Autodesk Inventor part; units mm, degrees
ref_plane "YZ Plane" through (0, 0, 0) normal (1, 0, 0) x (0, 1, 0)
ref_plane "XZ Plane" through (0, 0, 0) normal (0, 1, 0) x (-1, 0, 0)
ref_plane "XY Plane" through (0, 0, 0) normal (0, 0, 1) x (1, 0, 0)
sketch "Main Sketch" plane through (0, 0, 0) normal (0, 1, 0) x (-1, 0, 0)
  line L0 (-57.375, -12.0472) -> (-57.375, 12.0472)
  line L1 (-57.375, 12.0472) -> (47.625, -10) construction
  line L2 (47.625, 10) -> (-57.375, -12.0472) construction
  circle A0 centre (47.625, 0) radius 7
  arc A1 (47.625, -10) -> (47.625, 10) centre (47.625, 0) ccw
  line L3 (-40.875, 17.5) -> (-57.375, 17.5)
  line L4 (-57.375, 17.5) -> (-57.375, -17.5)
  line L5 (-57.375, -17.5) -> (-40.875, -17.5)
  line L6 (-40.875, 17.5) -> (-57.375, -17.5) construction
  line L7 (-57.375, 17.5) -> (-40.875, -17.5) construction
  line L8 (47.625, -10) -> (-40.875, -10)
  line L9 (-40.875, -17.5) -> (-40.875, -10)
  line L10 (-40.875, 10) -> (-40.875, 17.5)
  line L11 (-40.875, 10) -> (47.625, 10)
  point P0 (0, 0)
  point P1 (-49.125, 0)
  dimension "d3" = 14
  dimension "d4" = 105
  dimension "d13" = 16.5
  dimension "d14" = 35
  dimension "d15" = 0
  dimension "d18" = 20
extrude "Main Extrusion" add sketch "Main Sketch" along normal blind 4
sketch "Screw Holes Sketch" plane through (0, 4, 0) normal (0, 1, 0) x (1, 0, 0)
  circle A0 centre (46.125, -8.75) radius 2
  line L0 (57.375, 17.5) -> (40.875, 17.5)
  line L1 (40.875, -17.5) -> (57.375, -17.5)
  line L2 (35.2664, 0) -> (65.7891, 0)
  line L3 (51.375, -27.0398) -> (51.375, 30.2346) construction
  line L4 (57.375, -17.5) -> (57.375, 17.5)
  line L5 (40.875, -10) -> (40.875, -17.5)
  circle A1 centre (46.125, 8.75) radius 2
  line L6 (51.375, 27.0398) -> (51.375, -30.2346) construction
  point P0 (0, 0)
  dimension "d21" = 4
  dimension "d22" = 35
  dimension "d23" = 6
  dimension "d24" = 5.25
  dimension "d25" = 5.25
  dimension "d26" = 10.5
  dimension "d27" = 8.75
  dimension "d28" = 17.5
extrude "Screw Holes Cut" cut sketch "Screw Holes Sketch" against normal through all
fillet "Fillet1" radius 6 2 edges at (40.875, 2, -17.5) (40.875, 2, 17.5)
properties part number "TapeMeasureBracketSide"
CAD build for the part. Positions are in the model's coordinates, mm. A direction names the side the tool comes from. Coordinates: 2 decimals unless noted, no trailing zeros. Order: outer loops, then holes, each group sorted by start corner. A loop starts at its lowest first (then second) coordinate and runs counter-clockwise, first axis right, second up. Notation, with made-up numbers: (30, 36.5) -> (42, 36.5) arc R31 ccw to (42, 69.5) -> close; hole circle Ø3 at (38, -29). An arc over 180 degrees is marked (long way). Answer in a Markdown table with one row per item.
1) Which spindle directions (+Z, -Z, +X, -X, +Y, -Y) get a long thin tool onto all of the face, cutting with end or side? Do faces 1 (the face through (-3, 2, 10)), 2 (the face through (-4, 2, -10)), 3 (the face through (-54.302, 1.972, -2.103)). Say none if no direction does.
Check values:
| item | result |
|---|---|
| face 1 | +Z, -X, +Y, -Y |
| face 2 | -Z, -X, +Y, -Y |
| face 3 | +Y, -Y |
2) Band-saw the part on C-C (x = 18). List the corners of the cut face in (y, z).
Check values:
| item | result |
|---|---|
| outline | (0, -10) -> (4, -10) -> (4, 10) -> (0, 10) -> close |
3) Band-saw the part on D-D (z = -8.75). List the corners of the cut face in (x, y) (3 decimals), and give its area (3 significant figures).
Check values:
| item | result |
|---|---|
| outline | (-52.466, 0) -> (44.125, 0) -> (44.125, 4) -> (-52.466, 4) -> close; (48.125, 0) -> (57.375, 0) -> (57.375, 4) -> (48.125, 4) -> close |
| area | 423 mm2 |
4) Band-saw the part on B-B (z = 0). List the corners of the cut face in (x, y) (3 decimals).
Check values:
| item | result |
|---|---|
| outline | (-57.625, 0) -> (-54.625, 0) -> (-54.625, 4) -> (-57.625, 4) -> close; (-40.625, 0) -> (57.375, 0) -> (57.375, 4) -> (-40.625, 4) -> close |
5) Flat gauge pins, fed straight in: P1, Ø2, axis at y = 1, z = -1.5, coming from the -X side; P2, Ø1.5, axis at y = 2, z = 8, coming from the -X side; P3, Ø1.2, axis at y = 2.5, z = 11, coming from the -X side (3 decimals); P4, Ø3, axis at x = 46.125, z = -8.75, coming from the +Y side. Where does each tip first touch, or does it go through?
Check values:
| item | result |
|---|---|
| P1 | x = -57.61 |
| P2 | x = -54.51 |
| P3 | x = 40.875 |
| P4 | through |
6) Band-saw the part on A-A (y = 0.95). List the corners of the cut face in (x, z) (3 decimals).
Check values:
| item | result |
|---|---|
| outline | (-47.625, -10) -> (40.875, -10) -> (40.875, -11.5) arc R6 ccw to (46.875, -17.5) -> (57.375, -17.5) -> (57.375, 17.5) -> (46.875, 17.5) arc R6 ccw to (40.875, 11.5) -> (40.875, 10) -> (-47.625, 10) arc R10 ccw to start; hole circle Ø14 at (-47.625, 0); hole circle Ø4 at (46.125, -8.75); hole circle Ø4 at (46.125, 8.75) |
7) Drill centre lines: line 1 (Z direction, x = 8.5, y = 0.6); line 2 (Z direction, x = -44, y = 3.3); line 3 (X direction, y = 1.55, z = -8.75) (3 decimals). Where is each one in solid material? Low to high.
Check values:
| item | result |
|---|---|
| line 1 | -10 to 10 |
| line 2 | -10 to -5.99, 5.99 to 10 |
| line 3 | -52.466 to 44.125, 48.125 to 57.375 |
8) Mould opens along Z. For faces 4 (the face through (44.65, 2.03, -10.1)), 5 (the face through (57.375, 2, 0)), 6 (the face through (-57.623, 1.972, 0.22)) say: pulls with the +Z half, pulls with the -Z half, needs draft (parallel to the pull), parting line crosses it, or undercut.
Check values:
| item | result |
|---|---|
| face 4 | undercut |
| face 5 | needs draft |
| face 6 | parting line crosses it |
